Read the model definition and answer for the solid it produces. Units are mm, in the model's axes. A direction names the side the tool comes from. Coordinates: 2 decimals unless noted, no trailing zeros. Order: outer loops, then holes, each group sorted by start corner. A loop starts at its lowest first (then second) coordinate and runs counter-clockwise, first axis right, second up.
from build123d import *

# Parameters (mm, degrees)
F2_W     = 8.4896776825
F2_H     = 8.0091296695
F3_DEPTH = 6.35


with BuildPart() as f1:
    # F0 (on Front) → F1 (revolve)
    with BuildSketch(Plane.XZ):
        with BuildLine():
            Line((-24.7842427343, 0), (0, 0))
            Line((0, 0), (0, 56.3033334911))
            Line((0, 56.3033334911), (-24.7842427343, 56.3033334911))
            Line((-24.7842427343, 56.3033334911), (-24.7842427343, 44.3374402821))
            Line((-24.7842427343, 44.3374402821), (-22.8732544929, 44.3628020585))
            ThreePointArc((-22.8732544929, 44.3628020585), (-20.6233794189, 38.6463349976), (-15.6248472631, 35.0749753416))
            Line((-15.6248472631, 35.0749753416), (-15.6248472631, 16.4330303669))
            ThreePointArc((-15.6248472631, 16.4330303669), (-22.330766473, 12.4969846373), (-24.7842427343, 5.1184846088))
            Line((-24.7842427343, 5.1184846088), (-24.7842427343, 0))
        make_face()
    revolve(axis=Axis((0, 0, 28.1516667455), (0, 0, 1)))

    # F2 (on face) → F3 (cut)
    with BuildSketch(Plane.XY.offset(56.3033334911)):
        with BuildLine():
            Line((4.0728570893, 25.9603485465), (-4.4168205932, 25.9603485465))
            Line((-4.4168205932, 25.9603485465), (-4.4168205932, 17.2965058223))
            ThreePointArc((-4.4168205932, 17.2965058223), (-0.1770607755, 17.8506601361), (4.0728570893, 17.3807149721))
            Line((4.0728570893, 17.3807149721), (4.0728570893, 25.9603485465))
        make_face()
        with BuildLine():
            ThreePointArc((4.0728570893, 17.3807149721), (-0.1770607755, 17.8506601361), (-4.4168205932, 17.2965058223))
            Line((-4.4168205932, 17.2965058223), (-4.4168205932, 3.8551511243))
            Line((-4.4168205932, 3.8551511243), (4.0728570893, 3.8551511243))
            Line((4.0728570893, 3.8551511243), (4.0728570893, 17.3807149721))
        make_face()
        with BuildLine():
            Line((-4.4168205932, 3.8551511243), (-4.4168205932, 17.2965058223))
            ThreePointArc((-4.4168205932, 17.2965058223), (-12.8254291429, 12.4171568852), (-17.4302962574, 3.8551511243))
            Line((-17.4302962574, 3.8551511243), (-4.4168205932, 3.8551511243))
        make_face()
        with BuildLine():
            ThreePointArc((17.4302962574, 3.8551511243), (12.7016384893, 12.5437553188), (4.0728570893, 17.3807149721))
            Line((4.0728570893, 17.3807149721), (4.0728570893, 3.8551511243))
            Line((4.0728570893, 3.8551511243), (17.4302962574, 3.8551511243))
        make_face()
        with BuildLine():
            Line((-4.4168205932, -4.1539785452), (-4.4168205932, 3.8551511243))
            Line((-4.4168205932, 3.8551511243), (-17.4302962574, 3.8551511243))
            ThreePointArc((-17.4302962574, 3.8551511243), (-17.8508798192, -0.153321532), (-17.3615056967, -4.1539785452))
            Line((-17.3615056967, -4.1539785452), (-4.4168205932, -4.1539785452))
        make_face()
        with BuildLine():
            ThreePointArc((-17.3615056967, -4.1539785452), (-17.8508798192, -0.153321532), (-17.4302962574, 3.8551511243))
            Line((-17.4302962574, 3.8551511243), (-28.2840281725, 3.8551511243))
            Line((-28.2840281725, 3.8551511243), (-28.2840281725, -4.1539785452))
            Line((-28.2840281725, -4.1539785452), (-17.3615056967, -4.1539785452))
        make_face()
        with BuildLine():
            Line((17.4302962574, 3.8551511243), (4.0728570893, 3.8551511243))
            Line((4.0728570893, 3.8551511243), (4.0728570893, -4.1539785452))
            Line((4.0728570893, -4.1539785452), (17.3615056967, -4.1539785452))
            ThreePointArc((17.3615056967, -4.1539785452), (17.7286068375, -2.0913912627), (17.8515382478, 0))
            ThreePointArc((17.8515382478, 0), (17.7459152782, 1.9390484139), (17.4302962574, 3.8551511243))
        make_face()
        with BuildLine():
            Line((30.1826205105, 3.8551511243), (17.4302962574, 3.8551511243))
            ThreePointArc((17.4302962574, 3.8551511243), (17.7459152782, 1.9390484139), (17.8515382478, 0))
            ThreePointArc((17.8515382478, 0), (17.7286068375, -2.0913912627), (17.3615056967, -4.1539785452))
            Line((17.3615056967, -4.1539785452), (30.1826205105, -4.1539785452))
            Line((30.1826205105, -4.1539785452), (30.1826205105, 3.8551511243))
        make_face()
        with BuildLine():
            Line((4.0728570893, -4.1539785452), (-4.4168205932, -4.1539785452))
            Line((-4.4168205932, -4.1539785452), (-4.4168205932, -17.2965058223))
            ThreePointArc((-4.4168205932, -17.2965058223), (-0.1770607755, -17.8506601361), (4.0728570893, -17.3807149721))
            Line((4.0728570893, -17.3807149721), (4.0728570893, -4.1539785452))
        make_face()
        with BuildLine():
            Line((-4.4168205932, -17.2965058223), (-4.4168205932, -4.1539785452))
            Line((-4.4168205932, -4.1539785452), (-17.3615056967, -4.1539785452))
            ThreePointArc((-17.3615056967, -4.1539785452), (-12.7183088422, -12.5268526777), (-4.4168205932, -17.2965058223))
        make_face()
        with BuildLine():
            Line((17.3615056967, -4.1539785452), (4.0728570893, -4.1539785452))
            Line((4.0728570893, -4.1539785452), (4.0728570893, -17.3807149721))
            ThreePointArc((4.0728570893, -17.3807149721), (12.5934354383, -12.6523832409), (17.3615056967, -4.1539785452))
        make_face()
        with BuildLine():
            ThreePointArc((4.0728570893, -17.3807149721), (-0.1770607755, -17.8506601361), (-4.4168205932, -17.2965058223))
            Line((-4.4168205932, -17.2965058223), (-4.4168205932, -27.8610046953))
            Line((-4.4168205932, -27.8610046953), (4.0728570893, -27.8610046953))
            Line((4.0728570893, -27.8610046953), (4.0728570893, -17.3807149721))
        make_face()
        with Locations((-0.1719817519, -0.1494137105)):
            Rectangle(F2_W, F2_H)
    extrude(amount=-F3_DEPTH, mode=Mode.SUBTRACT)


solid = f1.part
Q1. The part is cut by section A-A, the plane x = 0. Determine the outline of the cut face in (y, z), then the cut area to 3 significant figures.
Q2. The part is cut by section C-C, the plane z = 27.5. Determine the outline of the cut face in (x, y).
Q3. Which of the six approach directions +Z, -Z, +X, -X, +Y, -Y give full straight-line access (tool end or side, diameter ignored) to faces 4 (the cylindrical face through (11.516, -10.56, 25.624)), 5 (the flat face through (21, 3.855, 53)), 6 (the flat face through (4.073, 21, 53)), 7 (the cylindrical face through (-12.729, 12.516, 53.173))?
Q4. Determine the mould class of faces 1 (the cylindrical face through (-23.64, -7.44, 2.52)), 2 (the flat face through (14, 14, 56.303)), 3 (the cylindrical face through (12.495, -12.749, 53.173)) for opening direction Y: +Y half, -Y half, draft (parallel to the pull), parting line (faces both ways), or undercut.
Q5. Each of these flat-tipped pins is pushed along its axis until it touches: P1, Ø3, axis at x = -20, z = 53.5, coming from the -Y side; P2, Ø12, axis at y = 13.5, z = 45, coming from the -X side; P3, Ø7, axis at x = 21.5, z = 51.5, coming from the +Y side. Where does it stop, or does it pass through?
Q6. Straight lines are drawn through the part: L1, parallel to Z at x = 4.5, y = -15; L2, parallel to Z at x = -5, y = 0.5; L3, parallel to Z at x = -18, y = 8. For each, find the intervals that lie inside material, in ascending order.
Q7. The part is cut by section D-D, the plane z = 12. Determine the outline of the cut face in (x, y).
Computed values:
1. outline: (-24.78, 0) - (24.78, 0) - (24.78, 5.12) arc R11.05 ccw to (15.62, 16.43) - (15.62, 35.07) arc R10.82 ccw to (22.87, 44.36) - (24.78, 44.34) - (24.78, 49.95) - (-24.78, 49.95) - (-24.78, 44.34) - (-22.87, 44.36) arc R10.82 ccw to (-15.62, 35.07) - (-15.62, 16.43) arc R11.05 ccw to (-24.78, 5.12) - close
1. area: 2,010 mm2
2. outline: circle Ø31.25 at (0, 0)
3. face 4: none
3. face 5: +Z, +X, -X
3. face 6: +Z, +Y, -Y
3. face 7: +Z
4. face 1: parting line
4. face 2: draft
4. face 3: undercut
5. P1: stops at y = -16.49
5. P2: stops at x = -23.62
5. P3: stops at y = 17.04
6. L1: z = 0 to 16.43, 35.09 to 49.95
6. L2: z = 0 to 49.95
6. L3: z = 0 to 14.85, 37.61 to 56.3
7. outline: circle Ø45.42 at (0, 0)
